```python
from build123d import *

# Parameters (mm, degrees)
SKETCH_1_W          = 25
SKETCH_1_H          = 34
SKETCH_1_H_2        = 108
EXTRUDE_1_DEPTH     = 3
SKETCH_2_R          = 2.05
SKETCH_2_R_2        = 1.55
CUT_EXTRUDE_1_DEPTH = 10
SKETCH_3_R          = 1.55
CUT_EXTRUDE_2_DEPTH = 10
FILLET_1_R          = 8
SKETCH_4_R          = 4
CUT_EXTRUDE_4_DEPTH = 10


with BuildPart() as part:
    # 草图1 → 凸台-拉伸1 (new body)
    with BuildSketch(Plane(origin=(0, 0, 0), x_dir=(1, 0, 0), z_dir=(0, 1, 0))):
        with Locations((-25, 0)):
            Rectangle(SKETCH_1_W, SKETCH_1_H)
        with Locations((0, 71)):
            Rectangle(SKETCH_1_W, SKETCH_1_H_2)
        Rectangle(SKETCH_1_W, SKETCH_1_H)
        with Locations((0, -71)):
            Rectangle(SKETCH_1_W, SKETCH_1_H_2)
    extrude(amount=EXTRUDE_1_DEPTH)

    # 草图2 → 切除-拉伸1 (cut)
    with BuildSketch(Plane(origin=(0, 0, 0), x_dir=(-1, 0, 0), z_dir=(0, -1, 0))):
        with Locations(Location((-1.25, -11.75, 0), (0, 0, 90))):
            Circle(SKETCH_2_R)
        with Locations(Location((-1.25, 11.75, 0), (0, 0, 90))):
            Circle(SKETCH_2_R)
        with Locations(Location((16.25, 11.75, 0), (0, 0, 90))):
            Circle(SKETCH_2_R)
        with Locations(Location((16.25, -11.75, 0), (0, 0, 90))):
            Circle(SKETCH_2_R)
        with Locations(Location((0, -115, 0), (0, 0, 90))):
            Circle(SKETCH_2_R_2)
        with Locations(Location((0, -67, 0), (0, 0, 90))):
            Circle(SKETCH_2_R_2)
        with Locations(Location((0, 115, 0), (0, 0, 270))):
            Circle(SKETCH_2_R_2)
        with Locations(Location((0, 67, 0), (0, 0, 270))):
            Circle(SKETCH_2_R_2)
    extrude(amount=-CUT_EXTRUDE_1_DEPTH, mode=Mode.SUBTRACT)

    # 草图3 → 切除-拉伸2 (cut)
    with BuildSketch(Plane(origin=(0, 0, 0), x_dir=(-1, 0, 0), z_dir=(0, -1, 0))):
        with Locations(Location((0.5, 83, 0), (0, 0, 90))):
            Circle(SKETCH_3_R)
        with Locations(Location((0.5, 103, 0), (0, 0, 90))):
            Circle(SKETCH_3_R)
    extrude(amount=-CUT_EXTRUDE_2_DEPTH, mode=Mode.SUBTRACT)

    # 圆角1
    fillet_1_edges = [part.edges().sort_by_distance(p)[0] for p in [
        (-37.5, 1.5, -17),
        (-12.5, 1.5, -17),
        (-12.5, 1.5, -125),
        (12.5, 1.5, -125),
        (12.5, 1.5, 125),
        (-12.5, 1.5, 125),
        (-12.5, 1.5, 17),
        (-37.5, 1.5, 17),
    ]]
    fillet(fillet_1_edges, radius=FILLET_1_R)

    # 草图4 → 切除-拉伸4 (cut)
    with BuildSketch(Plane(origin=(0, 0, 0), x_dir=(1, 0, 0), z_dir=(0, 1, 0))):
        with Locations(Location((0, -39, 0), (0, 0, 270))):
            Circle(SKETCH_4_R)
    extrude(amount=CUT_EXTRUDE_4_DEPTH, mode=Mode.SUBTRACT)


solid = part.part
```
Model file for the job. Use its own axes, mm. Coordinates: 2 decimals unless noted, no trailing zeros. Loops run counter-clockwise (first coordinate to the right, second up) from the corner with the lowest first, then second, coordinate; pieces in that order, holes last. Notation, with made-up numbers: (5, 16) - (25, 16) arc R18 ccw to (25, 44) - close; hole circle Ø1 at (-32, 2.5). An arc over 180 degrees is marked (long way). Answer as a JSON object with one key per item and string values. Group by question number.
(1) Cut at A-A (z = 39). Give the cut face in (x, y).
(2) Cut at D-D (x = -16.25). Give the cut face in (y, z), then the cut area to 3 significant figures.
(3) Cut at B-B (y = 2.2). State how many separate pieces and enclosed holes the cut face has, then the cut area to 3 significant figures.
(4) Probe line 1 along X through (y, z) = (1.85, -103); line 2 along X through (y, z) = (1.75, 11.75); line 3 along X through (y, z) = (1.9, 115). List the from-to ranges inside material, lowest first.
(5) Flat gauge pins, fed straight in: pin 1 (0.9 mm diameter, centred on y = 1.5, z = -92, fed in from -X); pin 2 (5 mm diameter, centred on x = 0, z = 39, fed in from -Y) (3 decimals); pin 3 (1.5 mm diameter, centred on x = -29.5, y = 1, fed in from -Z); pin 4 (0.9 mm diameter, centred on x = -23, y = 2, fed in from +Z). Where does each tip first touch, or does it go through?
(6) Cut at C-C (z = -11.75). Give the cut face in (x, y), then the cut area to 3 significant figures.
(7) Two-plate mould, pull along X, no slides. Class faces 1 (the face through (10.094, 1.521, -122.719)), 2 (the face through (-2, 0, -2)), 3 (the face through (-10.219, 1.521, -122.594)), 4 (the face through (-16.2, 1.5, -9.7)): released by +X, released by -X, zero draft, split by the parting line, or undercut.
Geometry says:
{
 "1": {"outline": "(-12.5, 0) - (-4, 0) - (-4, 3) - (-12.5, 3) - close; (4, 0) - (12.5, 0) - (12.5, 3) - (4, 3) - close"},
 "2": {"outline": "(0, -18.22) - (3, -18.22) - (3, -13.8) - (0, -13.8) - close; (0, -9.7) - (3, -9.7) - (3, 9.7) - (0, 9.7) - close; (0, 13.8) - (3, 13.8) - (3, 18.22) - (0, 18.22) - close", "area": "84.7 mm^2"},
 "3": {"separate pieces": "1", "enclosed holes": "11", "area": "6,900 mm^2"},
 "4": {"line 1": "x = -12.5 to -2.05, 1.05 to 12.5", "line 2": "x = -37.01 to -18.3, -14.2 to -0.8, 3.3 to 12.5", "line 3": "x = -12.5 to -1.55, 1.55 to 12.5"},
 "5": {"pin 1": "stops at x = -12.5", "pin 2": "passes through", "pin 3": "stops at z = -17", "pin 4": "stops at z = 17"},
 "6": {"outline": "(-37.01, 0) - (-18.3, 0) - (-18.3, 3) - (-37.01, 3) - close; (-14.2, 0) - (-0.8, 0) - (-0.8, 3) - (-14.2, 3) - close; (3.3, 0) - (12.5, 0) - (12.5, 3) - (3.3, 3) - close", "area": "124 mm^2"},
 "7": {"face 1": "released by +X", "face 2": "zero draft", "face 3": "released by -X", "face 4": "undercut"}
}
